Can you work these out from the model? Positions are in its coordinate system, mm. Give positions to 0.01 mm unless a question says otherwise; leave off trailing zeros.
```python
from build123d import *

# Parameters (mm, degrees)
ESQUISSE1_R                       = 10
ESQUISSE1_R_2                     = 8
EXTRUSION1_REACH                  = 433.016
EXTRUSION1_END_RADIUS             = 8
ESQUISSE3_R                       = 2
EXTRUSION1_DIRECTION_2_REACH      = 433.016
EXTRUSION1_DIRECTION_2_END_RADIUS = 8


with BuildPart() as part:
    # Balayage1: sweep along a curve in space
    with BuildLine() as balayage1_path:
        Line((0, 0, 0), (12.990381057, -7.5, 0))
        Line((0, 0, 0), (-10.26979763, 5.929270426, 0))
        ThreePointArc((-23.243938294, 14.727794485, 2.973935241), (-17.035828208, 10.165933144, 0.751028422), (-10.26979763, 5.929270426, 0))
        Line((-23.243938294, 14.727794485, 2.973935241), (-86.480363257, 65.200039483, 34.722605481))
        ThreePointArc((-106.469208033, 73.428950509, 40.880198038), (-95.752548684, 70.629649492, 38.3883833), (-86.480363257, 65.200039483, 34.722605481))
        Line((-106.469208033, 73.428950509, 40.880198038), (-400, 110, 89))
    # Esquisse1 → Balayage1 (sweep)
    with BuildSketch(Plane(origin=(-400, 110, 89), x_dir=(0.15933409799773637, -0.019851461389881916, 0.9870251084425026), z_dir=(-0.9794525040369775, 0.12203014804395138, 0.1605659842683569))):
        Circle(ESQUISSE1_R)
        Circle(ESQUISSE1_R_2, mode=Mode.SUBTRACT)
    sweep(path=balayage1_path.line)

    # Extrusion1: up to this cylinder (the profile starts inside it)
    extrusion1_end = Plane(origin=(6.062177957, -3.500000075, 0), z_dir=(0.866025403784438, -0.500000000000001, 0)) * Cylinder(EXTRUSION1_END_RADIUS, 883.032, mode=Mode.PRIVATE)
    # Esquisse3 → Extrusion1 (add, up to the surface)
    with BuildSketch(Plane.XY, mode=Mode.PRIVATE) as extrusion1_sk1:
        with Locations((6.062177826, -3.5)):
            Circle(ESQUISSE3_R)
    extrusion1_tool1 = extrude(extrusion1_sk1.sketch, amount=EXTRUSION1_REACH, mode=Mode.PRIVATE) & extrusion1_end
    add(extrusion1_tool1.solids().sort_by_distance((6.062178, -3.5, 0))[0])

    # Extrusion1 direction 2: up to this cylinder (the profile starts inside it)
    extrusion1_direction_2_end = Plane(origin=(6.062177957, -3.500000075, 0), z_dir=(0.866025403784438, -0.500000000000001, 0)) * Cylinder(EXTRUSION1_DIRECTION_2_END_RADIUS, 883.032, mode=Mode.PRIVATE)
    # Esquisse3 → Extrusion1 direction 2 (add, up to the surface)
    with BuildSketch(Plane.XY, mode=Mode.PRIVATE) as extrusion1_direction_2_sk1:
        with Locations((6.062177826, -3.5)):
            Circle(ESQUISSE3_R)
    extrusion1_direction_2_tool1 = extrude(extrusion1_direction_2_sk1.sketch, amount=-EXTRUSION1_DIRECTION_2_REACH, mode=Mode.PRIVATE) & extrusion1_direction_2_end
    add(extrusion1_direction_2_tool1.solids().sort_by_distance((6.062178, -3.5, 0))[0])


solid = part.part
```
1) Please list where these lines run through material, in increasing order: L1, parallel to Z at x = -85.5, y = 58.5; L2, parallel to Y at x = -208, z = 64; L3, parallel to X at y = 55, z = 28.
Values follow:
L1: z = 23.26 to 25.77, 39.79 to 42.31
L2: y = 78.46 to 81.36, 91.06 to 93.96
L3: x = -88.1 to -85.18, -61.87 to -58.96
2) If we mould it in two halves opening along X, with no side actions, what happens to faces 1 (the face through (-57.62, 40.2, 11.32)), 2 (the face through (13.014, -7.46, 8.195)), 3 (the face through (-400.98, 101.87, 89.21))? For each: +X half, -X half, draft (parallel to the pull), parting line (faces both ways), or undercut.
Values follow:
face 1: undercut
face 2: +X half
face 3: -X half
3) For pin 1 Ø10 at (x, y) = (-201, 91.5) entering from -Z; pin 2 Ø8 at (x, z) = (-290, 62.5) entering from -Y, each with a flat end and sliding along its axis, tell me the tip position at first contact or that it passes through.
Values follow:
pin 1: stops at z = 46.14
pin 2: stops at y = 87
